from build123d import *

# Parameters (mm, degrees)
SKETCH2_R           = 2.5
SKETCH2_R_2         = 1.25
BOSS_EXTRUDE2_DEPTH = 2.5


with BuildPart() as part:
    # Sketch2 → Boss-Extrude2 (new body)
    # profile 1 of 3: a face of its own
    with BuildSketch(Plane.XY):
        with BuildLine():
            Line((-12.5, 25), (-12.5, 45))
            ThreePointArc((-12.5, 45), (-15, 42.5), (-17.5, 45))
            Line((-17.5, 45), (-17.5, 20))
            Line((-17.5, 20), (-2.5, 20))
            Line((-2.5, 20), (-2.5, 0))
            ThreePointArc((-2.5, 0), (0, 2.5), (2.5, 0))
            Line((2.5, 0), (2.5, 25))
            Line((2.5, 25), (-12.5, 25))
        make_face()
    # profile 2 of 3: a face of its own
    with BuildSketch(Plane.XY):
        with Locations((-15, 45)):
            Circle(SKETCH2_R)
        with Locations((-15, 45)):
            Circle(SKETCH2_R_2, mode=Mode.SUBTRACT)
    # profile 3 of 3: a face of its own
    with BuildSketch(Plane.XY):
        Circle(SKETCH2_R)
        Circle(SKETCH2_R_2, mode=Mode.SUBTRACT)
    extrude(amount=BOSS_EXTRUDE2_DEPTH)


solid = part.part
Could you check a few things on this model? Use its own coordinates, in mm. A direction names the side the tool comes from. Round coordinates to 2 decimals unless told otherwise and drop trailing zeros. Loops run counter-clockwise (first coordinate to the right, second up) from the corner with the lowest first, then second, coordinate; pieces in that order, holes last. Notation, with made-up numbers: (-31.5, -23) -> (-10.5, -23) arc R18 cw to (-10.5, -1) -> close; hole circle Ø11 at (66, -15). An arc over 180 degrees is marked (long way). Use CSV: the item, a comma, the result in double quotes.
(1) If I drill on probe 1 along Y at (x, z) = (-15, 1.25); probe 2 along Y at (x, z) = (0, 1.1); probe 3 along Y at (x, z) = (-11.25, 1.05), over which ranges is the centre line in solid material (lowest first)? Write a range as [from, to].
Return value:
probe 1,"y = [20, 43.75], [46.25, 47.5]"
probe 2,"y = [-2.5, -1.25], [1.25, 25]"
probe 3,"y = [20, 25]"
(2) If we mould it in two halves opening along X, with no side actions, what happens to faces 1 (the cylindrical face through (-14.9, 47.5, 1.2)), 2 (the flat face through (-10, 20, 1)), 3 (the cylindrical face through (-0.27, -1.22, 1.23))? For each: +X half, -X half, draft (parallel to the pull), parting line (faces both ways), or undercut.
Return value:
face 1,"parting line"
face 2,"draft"
face 3,"undercut"
(3) Suppose I cut it at C-C on y = 38. Write out the boundary of the cut face in (x, z).
Return value:
outline,"(-17.5, 0) -> (-12.5, 0) -> (-12.5, 2.5) -> (-17.5, 2.5) -> close"
(4) Suppose I cut it at D-D on x = -9.75. Write out the boundary of the cut face in (y, z).
Return value:
outline,"(20, 0) -> (25, 0) -> (25, 2.5) -> (20, 2.5) -> close"
(5) Suppose I cut it at B-B on x = -15. Write out the boundary of the cut face in (y, z).
Return value:
outline,"(20, 0) -> (43.75, 0) -> (43.75, 2.5) -> (20, 2.5) -> close; (46.25, 0) -> (47.5, 0) -> (47.5, 2.5) -> (46.25, 2.5) -> close"
(6) For faces 4 (the flat face through (-2.5, 10, 1)), 5 (the cylindrical face through (-15.16, 46.24, 1.23)), 6 (the flat face through (-12.5, 35, 1)), which set-ups out of +Z, -Z, +X, -X, +Y, -Y let a thin tool reach every point of the face, with its end or its side?
Return value:
face 4,"+Z, -Z, -X, -Y"
face 5,"+Z, -Z"
face 6,"+Z, -Z, +X, +Y"
(7) Will these pins go through, and if not, where does the flat tip stop? pin 1 Ø1.2 at (y, z) = (35, 1) entering from +X; pin 2 Ø2 at (x, y) = (0, 0) entering from -Z; pin 3 Ø0.8 at (y, z) = (8.5, 1) entering from -X; pin 4 Ø1 at (x, z) = (-12, 2) entering from -Y.
Return value:
pin 1,"stops at x = -12.5"
pin 2,"passes through"
pin 3,"stops at x = -2.5"
pin 4,"stops at y = 20"
(8) Suppose I cut it at A-A on z = 2.05. Write out the boundary of the cut face in (x, y).
Return value:
outline,"(-17.5, 20) -> (-2.5, 20) -> (-2.5, 0) arc R2.5 ccw to (2.5, 0) -> (2.5, 25) -> (-12.5, 25) -> (-12.5, 45) arc R2.5 ccw to (-17.5, 45) -> close; hole circle Ø2.5 at (-15, 45); hole circle Ø2.5 at (0, 0)"
